Autodesk Inventor part; units mm, degrees
ref_plane "YZ Plane" through (0, 0, 0) normal (1, 0, 0) x (0, 1, 0)
ref_plane "XZ Plane" through (0, 0, 0) normal (0, 1, 0) x (-1, 0, 0)
ref_plane "XY Plane" through (0, 0, 0) normal (0, 0, 1) x (1, 0, 0)
sketch "Sketch1" plane through (0, 0, 0) normal (0, 1, 0) x (-1, 0, 0)
  circle A0 centre (0, 0) radius 264
  circle A1 centre (0, 0) radius 335
  line L0 (335, 0) -> (264, 0)
  line L1 (-264, 0) -> (-335, 0)
  line L2 (0, 264) -> (0, 335)
  point P0 (299.5, 0)
  point P1 (-299.5, 0)
  point P2 (0, 299.5)
  dimension "d1" = 670
  dimension "d4" = 528
extrude "Extrusion1" add sketch "Sketch1" along normal blind 6 contours L0 A1 L1 A0 | A0 L2 A1 L0 | A0 L1 A1 L2
sketch "Sketch2" plane through (0, 0, 0) normal (0, -1, 0) x (1, 0, 0)
  circle A0 centre (0, 0) radius 335
  circle A1 centre (0, 0) radius 264
  circle A2 centre (48.4947, 306.1834) radius 11.5
  circle A3 centre (0, 0) radius 264
  line L0 (48.4947, 306.1834) -> (0, 0)
  point P0 (0, 264)
  point P1 (265, 0)
  dimension "d5" = 310
  dimension "d7" = 23
extrude "Cut1" cut sketch "Sketch2" against normal blind 6 contours A2
pattern_circular "Circular Pattern1" count 20 over 360 about axis through (0, 0, 0) along (0, 1, 0) of "Cut1"
equation "\"d9\" = Thickness"
equation "\"BendRadius\" = Thickness"
equation "\"BendReliefWidth\" = Thickness"
equation "\"BendReliefDepth\" = 0.5 * Thickness"
equation "\"CornerReliefSize\" = 4 * Thickness"
equation "\"MinimumRemnant\" = 2 * Thickness"
equation "\"TransitionRadius\" = BendRadius"
equation "\"JacobiRadiusSize\" = BendRadius"
equation "\"GapSize\" = Thickness"
equation "\"d8\" = Thickness"
properties part number "PNS-712 accses hatch flangeipt" material "Steel"
Input: part model. Units: mm. Frame: model coordinates. Give positions to 0.01 mm unless a question says otherwise; leave off trailing zeros. Order: outer loops, then holes, each group sorted by start corner. A loop starts at its lowest first (then second) coordinate and runs counter-clockwise, first axis right, second up.
Q1. Section B-B on x = 0. Output: boundary loops of the cut face in (y, z).
Checked values:
outline: (0, -335) - (6, -335) - (6, -264) - (0, -264) - close; (0, 264) - (6, 264) - (6, 335) - (0, 335) - close
Q2. Ray query, probe 1 along X at (y, z) = (1.7, -38); probe 2 along Z at (x, y) = (138.5, 3.3); probe 3 along Z at (x, y) = (-56.5, 3.25). Return the intervals inside material, ascending.
Checked values:
probe 1: x = -332.84 to -310.89, -301.48 to -261.25, 261.25 to 301.48, 310.89 to 332.84
probe 2: z = -305.03 to -287.49, -264.93 to -224.75, 224.75 to 264.93, 287.49 to 305.03
probe 3: z = -330.2 to -314.44, -297.93 to -257.88, 257.88 to 297.93, 314.44 to 330.2
Q3. Draft query along Z for faces 1 (the cylindrical face through (265.845, 2.958, 203.842)), 2 (the cylindrical face through (294.736, 2.958, 47.396)), 3 (the flat face through (-98, 0, -247)). Return one class per face: +Z half, -Z half, draft (parallel to the pull), parting line (faces both ways), or undercut.
Checked values:
face 1: parting line
face 2: undercut
face 3: draft
Q4. Section C-C on y = 1.8. State how many separate pieces and enclosed holes the cut face has, and give its area (3 significant figures).
Checked values:
separate pieces: 1
enclosed holes: 21
area: 125,000 mm2
Q5. Contact query for flat-ended pins moving along their axis: pin 1 Ø20.5 at (x, z) = (-48.49, 306.18) entering from -Y (3 decimals); pin 2 Ø3 at (x, y) = (47, 2) entering from -Z. Output: stop coordinate, or through.
Checked values:
pin 1: passes through
pin 2: stops at z = -331.9
Q6. Section A-A on z = 0. Output: boundary loops of the cut face in (x, y), and give its area (3 significant figures).
Checked values:
outline: (-335, 0) - (-264, 0) - (-264, 6) - (-335, 6) - close; (264, 0) - (335, 0) - (335, 6) - (264, 6) - close
area: 852 mm2
